Part print with two shaded views. Sizes in mm from the minimum x, y, z corner. Give positions to 0.01 mm unless a question says otherwise; leave off trailing zeros. Loops run counter-clockwise (first coordinate to the right, second up) from the corner with the lowest first, then second, coordinate; pieces in that order, holes last. Notation, with made-up numbers: M -38,47.25 L -28,47.25 A29 ccw -28,80.25 Z; hole C -28.75,-10 d2. An arc over 180 degrees is marked long. Answer in a Markdown table with one row per item.
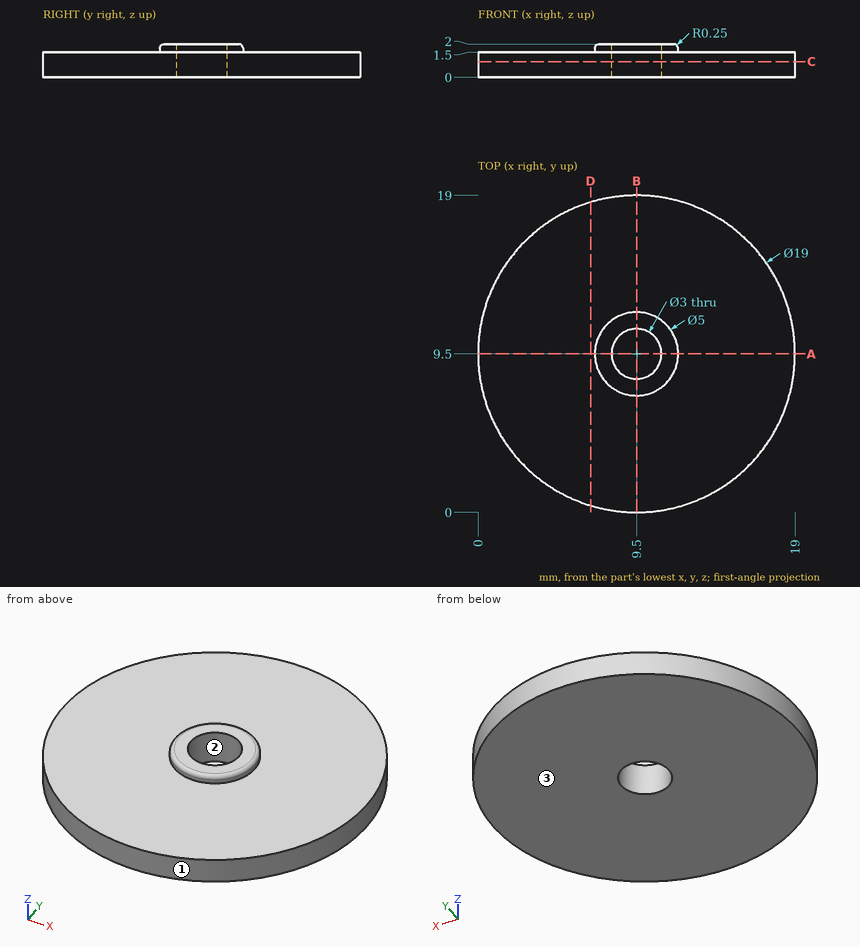
Q1. Mould opens along X. For the marked faces 1, 2 and 3 say: released by +X, released by -X, zero draft, split by the parting line, or undercut.
Reported:
| item | result |
|---|---|
| face 1 | split by the parting line |
| face 2 | undercut |
| face 3 | zero draft |
Q2. Saw through at C-C (z = 0.95). Give the cut face in (x, y), and give its area (3 significant figures).
Reported:
| item | result |
|---|---|
| outline | C 9.5,9.5 d19; hole C 9.5,9.5 d3 |
| area | 276 mm² |
Q3. Drop flat-ended pins along their axis: pin 1 (3 mm diameter, centred on x = 3, y = 12.5, fed in from +Z); pin 2 (2.5 mm diameter, centred on x = 9.5, y = 9.5, fed in from -Z); pin 3 (1 mm diameter, centred on x = 8, z = 1.5, fed in from -Y). Give the stop position or say it passes through.
Reported:
| item | result |
|---|---|
| pin 1 | z = 1.5 |
| pin 2 | through |
| pin 3 | y = 0.05 |
Q4. Probe probe 1 along Y at (x, z) = (9.5, 1.1); probe 2 along Y at (x, z) = (9.5, 1.65); probe 3 along Z at (x, y) = (10.25, 3). List the from-to ranges inside material, lowest first.
Reported:
| item | result |
|---|---|
| probe 1 | 0 to 8, 11 to 19 |
| probe 2 | 7 to 8, 11 to 12 |
| probe 3 | 0 to 1.5 |
Q5. Saw through at A-A (y = 9.5). Give the cut face in (x, z), and give its area (3 significant figures).
Reported:
| item | result |
|---|---|
| outline | M 0,0 L 8,0 L 8,2 L 7.25,2 A0.25 ccw 7,1.75 L 7,1.5 L 0,1.5 Z; M 11,0 L 19,0 L 19,1.5 L 12,1.5 L 12,1.75 A0.25 ccw 11.75,2 L 11,2 Z |
| area | 25.0 mm² |
Q6. Saw through at D-D (x = 6.75). Give the cut face in (y, z), and give its area (3 significant figures).
Reported:
| item | result |
|---|---|
| outline | M 0.41,0 L 18.59,0 L 18.59,1.5 L 0.41,1.5 Z |
| area | 27.3 mm² |
